```python
from build123d import *

# Parameters (mm, degrees)
F0_R     = 2.0955
F1_DEPTH = 12.7
F2_W     = 7.33298
F2_H     = 4.1894274764
F3_DEPTH = 2.0955
F4_R     = 2.284478014
F4_R_2   = 2.0955
F5_DEPTH = 5.08


# Not quite as in the source:
# - a fillet or chamfer that OpenCascade refuses, or shapes differently, is made with other operations: its cross-section is extruded or revolved along the edge and cut away or added


with BuildPart() as f1:
    # F0 (on Top) → F1 (new body)
    with BuildSketch(Plane.XY):
        Circle(F0_R)
    extrude(amount=F1_DEPTH)

    # F2 (on face) → F3 (join)
    with BuildSketch(Plane.XY.offset(12.7)):
        Rectangle(F2_W, F2_H)
    extrude(amount=F3_DEPTH)

    # F4 (on face) → F5 (join)
    with BuildSketch(Plane(origin=(0, 0, 0), x_dir=(1, 0, 0), z_dir=(0, 0, -1))):
        Circle(F4_R)
        Circle(F4_R_2, mode=Mode.SUBTRACT)
        Circle(F4_R_2)
    extrude(amount=F5_DEPTH)

    # F6: fillet of radius 1.5570711792 on 2 edges, made by hand

    # F6_s1 → F6_t2 (revolve, cut)
    with BuildSketch(Plane.XZ):
        with BuildLine():
            ThreePointArc((2.284478014, -0.7434996627), (2.2364941575, -0.3599294481), (2.0955, 0))
            Line((2.0955, 0), (2.284478014, 0))
            Line((2.284478014, 0), (2.284478014, -0.7434996627))
        make_face()
    revolve(axis=Axis((0, 0, 0), (0, 0, -1)), mode=Mode.SUBTRACT)

    # F6_s3 → F6_t4 (revolve, cut)
    with BuildSketch(Plane.XZ):
        with BuildLine():
            ThreePointArc((2.284478014, -3.5229288208), (1.8284224244, -4.6239444104), (0.7274068348, -5.08))
            Line((0.7274068348, -5.08), (2.284478014, -5.08))
            Line((2.284478014, -5.08), (2.284478014, -3.5229288208))
        make_face()
    revolve(axis=Axis((0, 0, -5.08), (0, 0, -1)), mode=Mode.SUBTRACT)


solid = f1.part
```
For this review, take the finished solid that the model builds, in its own axes (mm). A direction names the side the tool comes from. Round coordinates to 2 decimals unless told otherwise and drop trailing zeros. Order: outer loops, then holes, each group sorted by start corner. A loop starts at its lowest first (then second) coordinate and runs counter-clockwise, first axis right, second up.
Q1. Mouldability with a two-part tool opening along X and no side actions: class faces 4 (the cylindrical face through (-1.813, 1.39, -2.114)), 5 (the flat face through (-3.666, 0, 14)), 6 (the flat face through (0, 2.095, 14)) as pulls with the +X half, pulls with the -X half, needs draft (parallel to the pull), parting line crosses it, or undercut.
Findings below:
face 4: parting line crosses it
face 5: pulls with the -X half
face 6: needs draft
Q2. We need section B-B, the plane x = 2.5. Give the boundary of the cut face in (y, z).
Findings below:
outline: (-2.09, 12.7) - (2.09, 12.7) - (2.09, 14.8) - (-2.09, 14.8) - close
Q3. Insertion check: P1, Ø0.6, axis at x = 0, z = 13.5, coming from the -Y side; P2, Ø2, axis at x = 2.5, z = -1.5, coming from the -Y side; P3, Ø2, axis at x = 1, y = 1, coming from the -Z side; P4, Ø1.7, axis at x = -0.5, z = 13.5, coming from the +Y side. Each pin has a flat end and moves straight along its axis. Give the tip position at first contact, or say it passes through.
Findings below:
P1: stops at y = -2.09
P2: stops at y = -1.72
P3: stops at z = -5.08
P4: stops at y = 2.09
Q4. Wall thickness on line 1 (Y direction, x = -0.75, z = 13); line 2 (X direction, y = 0, z = 0.75); line 3 (Z direction, x = 3, y = -0.85): over which ranges is each line inside the solid? List them lowest first.
Findings below:
line 1: y = -2.09 to 2.09
line 2: x = -2.1 to 2.1
line 3: z = 12.7 to 14.8
Q5. We need section A-A, the plane z = 9. Give the boundary of the cut face in (x, y), plus the area to 3 significant figures.
Findings below:
outline: circle Ø4.19 at (0, 0)
area: 13.8 mm2
Q6. Machinability: for faces 1 (the cylindrical face through (2, 0.63, 6.26)), 2 (the flat face through (0, -2.095, 14)), 3 (the flat face through (0, 0, 14.795)), which of the approach directions +Z, -Z, +X, -X, +Y, -Y give a long, thin tool a straight path to every point of the face, cutting with its end or side? Answer none if there is none.
Findings below:
face 1: none
face 2: +Z, +X, -X, -Y
face 3: +Z, +X, -X, +Y, -Y
